from build123d import *

# Parameters (mm, degrees)
F0_W            = 10
F0_H            = 17
F2_R            = 3.5
F3_DEPTH        = 10.001
F3_COPIES_COUNT = 6
F5_DEPTH        = 10.001


# Not quite as in the source:
# - a pattern or mirror of a feature is missing from the dataset's text; its kind, count and spacing are read off the source's solid


with BuildPart() as f1:
    # F0 (on Front) → F1 (revolve)
    with BuildSketch(Plane.XZ):
        with Locations((5, 45.5)):
            Rectangle(F0_W, F0_H)
    revolve(axis=Axis((-28.7704151153, 0, 0), (-1, 0, 0)))

    # F2 (on face) → F3 (cut, through all)
    with BuildSketch(Plane(origin=(0, 0, 0), x_dir=(0, -1, 0), z_dir=(-1, 0, 0))):
        with Locations((41.5692193817, 24)):
            Circle(F2_R)
    f3 = extrude(amount=-F3_DEPTH, mode=Mode.SUBTRACT)

    # F3_copies: F3 ×6 about axis
    f3_copies_axis = Axis((0, 0, 0), (1, 0, 0))
    for i in range(1, F3_COPIES_COUNT):
        add(f3.rotate(f3_copies_axis, i * 360 / F3_COPIES_COUNT), mode=Mode.SUBTRACT)

    # F4 (on face) → F5 (cut, through all)
    with BuildSketch(Plane(origin=(0, 0, 0), x_dir=(0, -1, 0), z_dir=(-1, 0, 0))):
        with BuildLine():
            Line((-50, -20.3960780544), (-50, 20.3960780544))
            ThreePointArc((-50, 20.3960780544), (-54, 0), (-50, -20.3960780544))
        make_face()
        with BuildLine():
            ThreePointArc((54, 0), (52.990565198, 10.3923048454), (50, 20.3960780544))
            Line((50, 20.3960780544), (50, -20.3960780544))
            ThreePointArc((50, -20.3960780544), (52.990565198, -10.3923048454), (54, 0))
        make_face()
    extrude(amount=-F5_DEPTH, mode=Mode.SUBTRACT)


solid = f1.part
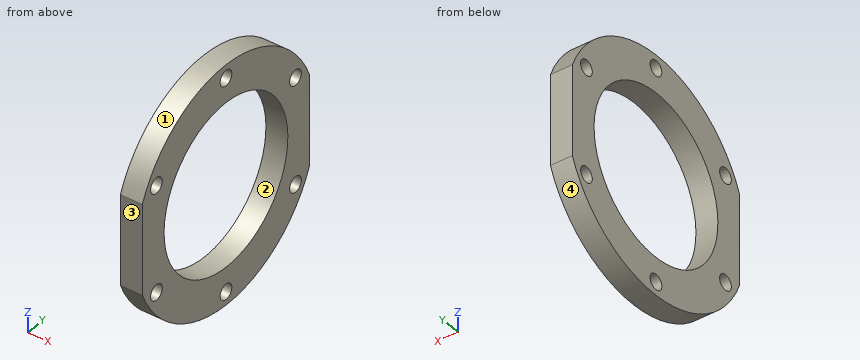
The listing builds one solid part. Answer for the finished solid, in the listing's coordinates (mm). Face numbers are marked on the shaded views. Coordinates: 2 decimals unless noted, no trailing zeros. Write each loop counter-clockwise with the first axis right and the second up, starting at its lowest first coordinate (ties: lowest second). Pieces come first, ordered by that corner, then holes. Notation, with made-up numbers: M 83,45.25 L 102,45.25 A24 ccw 102,82.25 Z; hole C 3.5,20.5 d4. An arc over 180 degrees is marked long. Use one line per item in the form item = value.
Item 1: Find section A-A, the plane y = 0. Give the vertices of the cut face in (x, z).
Model answer:
outline = M 0,-54 L 10,-54 L 10,-51.5 L 0,-51.5 Z; M 0,-44.5 L 10,-44.5 L 10,-37 L 0,-37 Z; M 0,37 L 10,37 L 10,44.5 L 0,44.5 Z; M 0,51.5 L 10,51.5 L 10,54 L 0,54 Z
Item 2: Find the intervals of material crossed by probe 1 along Y at (x, z) = (9.5, 26.5); probe 2 along Y at (x, z) = (4.5, -24); probe 3 along Z at (x, y) = (0.75, 44), in increasing order.
Model answer:
probe_1 = -47.05 to -44.02, -39.12 to -25.82, 25.82 to 39.12, 44.02 to 47.05
probe_2 = -48.37 to -45.07, -38.07 to -28.16, 28.16 to 38.07, 45.07 to 48.37
probe_3 = -31.3 to -26.52, -21.48 to 21.48, 26.52 to 31.3
Item 3: Find section C-C, the plane x = 3. Give the vertices of the cut face in (y, z), plus the area to 3 significant figures.
Model answer:
outline = M -50,-20.4 A54 ccw 50,-20.4 L 50,20.4 A54 ccw -50,20.4 Z; hole C -41.57,-24 d7; hole C -41.57,24 d7; hole C 0,0 d74; hole C 0,-48 d7; hole C 0,48 d7; hole C 41.57,-24 d7; hole C 41.57,24 d7
area = 4,410 mm2
Item 4: Find section B-B, the plane z = 0. Give the vertices of the cut face in (x, y), plus the area to 3 significant figures.
Model answer:
outline = M 0,-50 L 10,-50 L 10,-37 L 0,-37 Z; M 0,37 L 10,37 L 10,50 L 0,50 Z
area = 260 mm2
Item 5: The mould has two halves that part along Z. Classify the marked faces 1, 2, 3 and 4: released by +Z, released by -Z, zero draft, split by the parting line, or undercut.
Model answer:
face_1 = released by +Z
face_2 = undercut
face_3 = zero draft
face_4 = released by -Z
Item 6: Find section D-D, the plane y = -31. Give the vertices of the cut face in (x, z).
Model answer:
outline = M 0,-44.22 L 10,-44.22 L 10,-20.2 L 0,-20.2 Z; M 0,20.2 L 10,20.2 L 10,44.22 L 0,44.22 Z
Item 7: Given P1, Ø5.5, axis at y = 0, z = -48, coming from the +X side; P2, Ø1.5, axis at x = 5.5, y = 6, coming from the -Z side; P3, Ø2, axis at x = 7, y = -35.5, coming from the +Z side, each flat-ended and moving along its own axis, determine where each tip first touches the part or whether it passes through.
Model answer:
P1 = through
P2 = -53.74
P3 = 41.54
